from build123d import *

# Parameters (mm, degrees)
SKETCH1_W           = 30
SKETCH1_H           = 30
BOSS_EXTRUDE1_DEPTH = 4
SKETCH2_W           = 25
SKETCH2_H           = 25
BOSS_EXTRUDE2_DEPTH = 51
SKETCH3_R           = 3
BOSS_EXTRUDE3_DEPTH = 20


with BuildPart() as part:
    # Sketch1 → Boss-Extrude1 (new body)
    with BuildSketch(Plane.XY):
        Rectangle(SKETCH1_W, SKETCH1_H)
    extrude(amount=BOSS_EXTRUDE1_DEPTH)

    # Sketch2 → Boss-Extrude2 (add)
    with BuildSketch(Plane.XY.offset(4)):
        Rectangle(SKETCH2_W, SKETCH2_H)
    extrude(amount=BOSS_EXTRUDE2_DEPTH)

    # Sketch3 → Boss-Extrude3 (add)
    with BuildSketch(Plane.XY.offset(55)):
        Circle(SKETCH3_R)
    extrude(amount=BOSS_EXTRUDE3_DEPTH)


solid = part.part
The listing builds one solid part. Answer for the finished solid, in the listing's coordinates (mm). A direction names the side the tool comes from. Coordinates: 2 decimals unless noted, no trailing zeros. Write each loop counter-clockwise with the first axis right and the second up, starting at its lowest first coordinate (ties: lowest second). Pieces come first, ordered by that corner, then holes. Notation, with made-up numbers: M 14.25,-37.75 L 54.25,-37.75 A5 ccw 54.25,-32.75 Z; hole C -20,81.25 d1. An arc over 180 degrees is marked long. Write each question's results on one line, items separated by ' | '.
Item 1: The part is cut by section A-A on y = -10.25. Determine the outline of the cut face in (x, z).
Answer below:
outline: M -15,0 L 15,0 L 15,4 L 12.5,4 L 12.5,55 L -12.5,55 L -12.5,4 L -15,4 Z
Item 2: Which of the six approach directions +Z, -Z, +X, -X, +Y, -Y give full straight-line access (tool end or side, diameter ignored) to faces 1 (the face through (-12.5, 0, 29)), 2 (the face through (0, -12.5, 29)), 3 (the face through (-3, 0, 65))?
Answer below:
face 1: +Z, -X, +Y, -Y | face 2: +Z, +X, -X, -Y | face 3: +Z
Item 3: Consider probe 1 along Z at (x, y) = (1, -7.5); probe 2 along Z at (x, y) = (12.75, 4); probe 3 along X at (y, z) = (9, 28). Determine where each line is inside the solid, lowest interval first. Write a range as [from, to].
Answer below:
probe 1: [0, 55] | probe 2: [0, 4] | probe 3: [-12.5, 12.5]
Item 4: The part is cut by section B-B on x = 0. Determine the outline of the cut face in (y, z).
Answer below:
outline: M -15,0 L 15,0 L 15,4 L 12.5,4 L 12.5,55 L 3,55 L 3,75 L -3,75 L -3,55 L -12.5,55 L -12.5,4 L -15,4 Z
Item 5: Given P1, Ø6, axis at x = 7.5, y = -8, coming from the +Z side; P2, Ø4, axis at x = 3, z = 21, coming from the -Y side; P3, Ø1, axis at y = 1.5, z = 37, coming from the +X side; P4, Ø10, axis at y = -9.5, z = 62.5, coming from the -X side, each flat-ended and moving along its own axis, determine where each tip first touches the part or whether it passes through.
Answer below:
P1: z = 55 | P2: y = -12.5 | P3: x = 12.5 | P4: through
